from build123d import *

# Parameters (mm, degrees)
SKETCH1_R           = 4
SKETCH1_R_2         = 1.15
BOSS_EXTRUDE1_DEPTH = 20
SKETCH2_R           = 1.25
CUT_EXTRUDE1_DEPTH  = 10


with BuildPart() as part:
    # Sketch1 → Boss-Extrude1 (new body)
    with BuildSketch(Plane.XY):
        Circle(SKETCH1_R)
        Circle(SKETCH1_R_2, mode=Mode.SUBTRACT)
    extrude(amount=BOSS_EXTRUDE1_DEPTH)

    # Sketch2 → Cut-Extrude1 (cut)
    with BuildSketch(Plane(origin=(0, 0, 0), x_dir=(1, 0, 0), z_dir=(0, 1, 0))):
        with Locations(Location((0, -8.5, 0), (0, 0, 270))):
            Circle(SKETCH2_R)
    extrude(amount=-CUT_EXTRUDE1_DEPTH, mode=Mode.SUBTRACT)


solid = part.part
For this review, take the finished solid that the model builds, in its own axes (mm). Coordinates: 2 decimals unless noted, no trailing zeros. Order: outer loops, then holes, each group sorted by start corner. A loop starts at its lowest first (then second) coordinate and runs counter-clockwise, first axis right, second up. Notation, with made-up numbers: (23.5, -2) -> (66.5, -2) arc R28 cw to (66.5, 29) -> close; hole circle Ø2 at (61.25, -0.5). An arc over 180 degrees is marked (long way). Return JSON: item names as keys, results as strings.
1. We need section C-C on y = -3. Write out the cut boundary in (x, z), and give its area (3 significant figures).
Answer block:
{"outline": "(-2.65, 0) -> (2.65, 0) -> (2.65, 20) -> (-2.65, 20) -> close; hole circle Ø2.5 at (0, 8.5)", "area": "101 mm²"}
2. The part is to be moulded in two halves that separate along X. For faces 1 (the cylindrical face through (2.15, 3.373, 9.86)), 2 (the cylindrical face through (-1.109, -2.419, 9.077)), 3 (the flat face through (1, -1, 0)), say which applies: +X half, -X half, draft (parallel to the pull), parting line (faces both ways), or undercut.
Answer block:
{"face 1": "parting line", "face 2": "undercut", "face 3": "draft"}
3. We need section B-B on z = 12.5. Write out the cut boundary in (x, y), and give its area (3 significant figures).
Answer block:
{"outline": "circle Ø8 at (0, 0); hole circle Ø2.3 at (0, 0)", "area": "46.1 mm²"}
4. We need section D-D on x = 3. Write out the cut boundary in (y, z), and give its area (3 significant figures).
Answer block:
{"outline": "(-2.65, 0) -> (2.65, 0) -> (2.65, 20) -> (-2.65, 20) -> close", "area": "106 mm²"}
5. For line 1 (Z direction, x = 0, y = -3); line 2 (Y direction, x = 0, z = 13.5); line 3 (X direction, y = -2.35, z = 8.5), list the stretches that pass through material, from the lowest coordinate up. Write a range as from..to.
Answer block:
{"line 1": "0..7.25, 9.75..20", "line 2": "-4..-1.15, 1.15..4", "line 3": "-3.24..-1.25, 1.25..3.24"}
6. We need section A-A on x = 0.75. Write out the cut boundary in (y, z).
Answer block:
{"outline": "(-3.93, 0) -> (-0.87, 0) -> (-0.87, 7.5) -> (-3.93, 7.5) -> close; (-3.93, 9.5) -> (-0.87, 9.5) -> (-0.87, 20) -> (-3.93, 20) -> close; (0.87, 0) -> (3.93, 0) -> (3.93, 20) -> (0.87, 20) -> close"}
7. For pin 1 Ø1 at (y, z) = (3, 2.5) entering from +X; pin 2 Ø3 at (x, y) = (0, 0) entering from +Z; pin 3 Ø2 at (x, z) = (-3, 2) entering from +Y, all flat-tipped, find the tip position at first contact; note any pin that passes through.
Answer block:
{"pin 1": "x = 3.12", "pin 2": "z = 20", "pin 3": "y = 3.46"}
